Model file for the job. Use its own axes, mm. Round coordinates to 2 decimals unless told otherwise and drop trailing zeros. Order: outer loops, then holes, each group sorted by start corner. A loop starts at its lowest first (then second) coordinate and runs counter-clockwise, first axis right, second up. Notation, with made-up numbers: (5, 22) -> (33, 22) arc R18 cw to (33, 39) -> close; hole circle Ø8 at (-25, 1). An arc over 180 degrees is marked (long way). Answer as CSV lines item,"result".
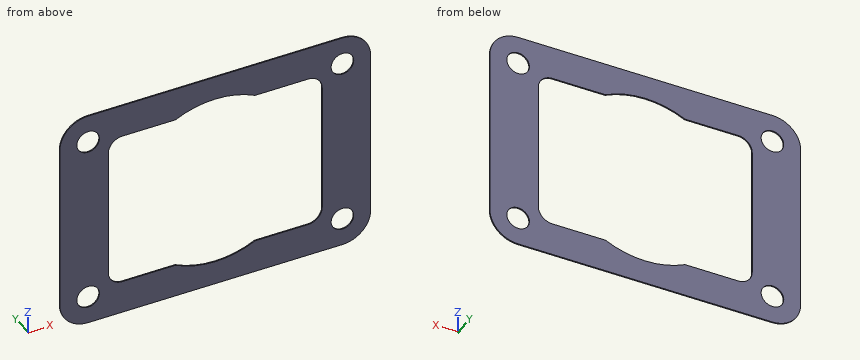
```python
from build123d import *

# Parameters (mm, degrees)
SKETCH1_W               = 139.7
SKETCH1_H               = 101.6
BOSS_EXTRUDE1_DEPTH     = 0.508
FILLET1_R               = 12.7
SKETCH2_W               = 96.139
SKETCH2_H               = 71.5772
CUT_EXTRUDE1_DEPTH      = 87.370831674
FILLET2_R               = 6.35
SKETCH3_R               = 5.08
CUT_EXTRUDE2_DEPTH      = 87.370831674
MIRROR2_COPY_1_SKETCH_R = 5.08
MIRROR2_COPY_1_DEPTH    = 87.370831674
SKETCH4_R               = 40.005
CUT_EXTRUDE3_DEPTH      = 87.370831674


with BuildPart() as part:
    # Sketch1 → Boss-Extrude1 (new body)
    with BuildSketch(Plane(origin=(0, 0, 0), x_dir=(1, 0, 0), z_dir=(0, 1, 0))):
        Rectangle(SKETCH1_W, SKETCH1_H)
    extrude(amount=BOSS_EXTRUDE1_DEPTH)

    # Fillet1
    fillet1_edges = [part.edges().sort_by_distance(p)[0] for p in [
        (-69.85, 0.254, -50.8),
        (69.85, 0.254, -50.8),
        (69.85, 0.254, 50.8),
        (-69.85, 0.254, 50.8),
    ]]
    fillet(fillet1_edges, radius=FILLET1_R)

    # Sketch2 → Cut-Extrude1 (cut, through all)
    with BuildSketch(Plane(origin=(0, 0.508, 0), x_dir=(1, 0, 0), z_dir=(0, 1, 0))):
        Rectangle(SKETCH2_W, SKETCH2_H)
    extrude(amount=-CUT_EXTRUDE1_DEPTH, mode=Mode.SUBTRACT)

    # Fillet2
    fillet2_edges = [part.edges().sort_by_distance(p)[0] for p in [
        (-48.0695, 0.254, 35.7886),
        (-48.0695, 0.254, -35.7886),
        (48.0695, 0.254, -35.7886),
        (48.0695, 0.254, 35.7886),
    ]]
    fillet(fillet2_edges, radius=FILLET2_R)

    # Sketch3 → Cut-Extrude2 (cut, through all)
    with BuildSketch(Plane(origin=(0, 0.508, 0), x_dir=(1, 0, 0), z_dir=(0, 1, 0))):
        with Locations(Location((-57.15, 38.1, 0), (0, 0, 270))):
            Circle(SKETCH3_R)
    cut_extrude2 = extrude(amount=-CUT_EXTRUDE2_DEPTH, mode=Mode.SUBTRACT)

    # Mirror1: Cut-Extrude2 across plane
    add(cut_extrude2.mirror(Plane(origin=(0, 0, 0), x_dir=(0, 0, 1), z_dir=(1, 0, 0))), mode=Mode.SUBTRACT)

    # Mirror2: Cut-Extrude2 across plane
    add(cut_extrude2.mirror(Plane.XY), mode=Mode.SUBTRACT)

    # Mirror2 copy 1 sketch → Mirror2 copy 1 (cut, through all)
    with BuildSketch(Plane(origin=(0, 0.508, 0), x_dir=(-1, 0, 0), z_dir=(0, 1, 0))):
        with Locations(Location((-57.15, 38.1, 0), (0, 0, 270))):
            Circle(MIRROR2_COPY_1_SKETCH_R)
    extrude(amount=-MIRROR2_COPY_1_DEPTH, mode=Mode.SUBTRACT)

    # Sketch4 → Cut-Extrude3 (cut, through all)
    with BuildSketch(Plane(origin=(0, 0.508, 0), x_dir=(1, 0, 0), z_dir=(0, 1, 0))):
        Circle(SKETCH4_R)
    extrude(amount=-CUT_EXTRUDE3_DEPTH, mode=Mode.SUBTRACT)


solid = part.part
```
Q1. Saw through at B-B (y = 0.1). State how many separate pieces and enclosed holes the cut face has, plus the area to 3 significant figures.
Checks:
separate pieces,"1"
enclosed holes,"5"
area,"6,680 mm²"
Q2. Saw through at C-C (x = 27.5). Write the cut outline in (y, z), plus the area to 3 significant figures.
Checks:
outline,"(0, -50.8) -> (0.51, -50.8) -> (0.51, -35.79) -> (0, -35.79) -> close; (0, 35.79) -> (0.51, 35.79) -> (0.51, 50.8) -> (0, 50.8) -> close"
area,"15.3 mm²"
Q3. Saw through at D-D (x = -59). Write the cut outline in (y, z), plus the area to 3 significant figures.
Checks:
outline,"(0, -50.66) -> (0.51, -50.66) -> (0.51, -42.83) -> (0, -42.83) -> close; (0, -33.37) -> (0.51, -33.37) -> (0.51, 33.37) -> (0, 33.37) -> close; (0, 42.83) -> (0.51, 42.83) -> (0.51, 50.66) -> (0, 50.66) -> close"
area,"41.9 mm²"
Q4. Flat gauge pin, fed straight in: pin 1 (9 mm diameter, centred on x = 57.15, z = 38.1, fed in from -Y). Where does the tip first touch, or does it go through?
Checks:
pin 1,"through"
Q5. Wall check: L1, parallel to Z at x = 57.15, y = 0.25; L2, parallel to Z at x = 28, y = 0.2; L3, parallel to X at y = 0.1, z = -23.5. Give the ranges that are in metal, low to high. Write a range as [from, to].
Checks:
L1,"[-50.8, -43.18], [-33.02, 33.02], [43.18, 50.8]"
L2,"[-50.8, -35.79], [35.79, 50.8]"
L3,"[-69.85, -48.07], [48.07, 69.85]"
Q6. Saw through at A-A (z = 20). Write the cut outline in (x, y), plus the area to 3 significant figures.
Checks:
outline,"(-69.85, 0) -> (-48.07, 0) -> (-48.07, 0.51) -> (-69.85, 0.51) -> close; (48.07, 0) -> (69.85, 0) -> (69.85, 0.51) -> (48.07, 0.51) -> close"
area,"22.1 mm²"
